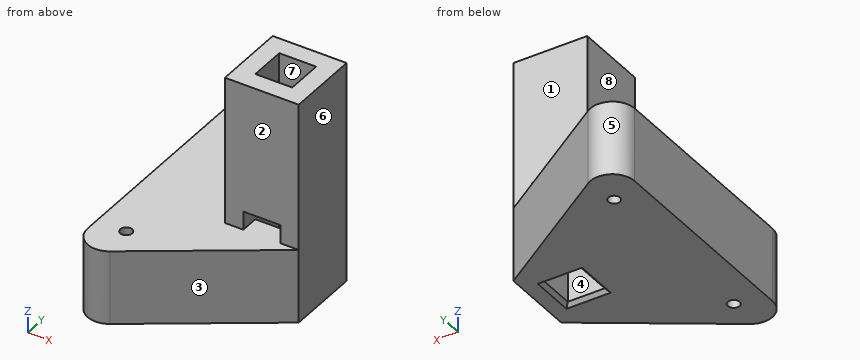
```python
from build123d import *

# Parameters (mm, degrees)
SKETCH_1_W          = 20
SKETCH_1_H          = 20
SKETCH_1_W_2        = 10
SKETCH_1_H_2        = 10
EXTRUDE_1_DEPTH     = 60
SKETCH_2_W          = 10
SKETCH_2_H          = 5
CUT_EXTRUDE_1_DEPTH = 80
SKETCH_4_R          = 1.6
EXTRUDE_3_DEPTH     = 20
CHAMFER_1_SIZE      = 1


with BuildPart() as part:
    # 草图1 → 凸台-拉伸1 (new body)
    with BuildSketch(Plane.XY):
        with Locations((5, 5)):
            Rectangle(SKETCH_1_W, SKETCH_1_H)
        with Locations((5, 5)):
            Rectangle(SKETCH_1_W_2, SKETCH_1_H_2, mode=Mode.SUBTRACT)
    extrude(amount=EXTRUDE_1_DEPTH)

    # 草图2 → 切除-拉伸1 (cut)
    with BuildSketch(Plane(origin=(0, 15, 0), x_dir=(1, 0, 0), z_dir=(0, 1, 0))):
        with Locations((5, -22.5)):
            Rectangle(SKETCH_2_W, SKETCH_2_H)
    extrude(amount=-CUT_EXTRUDE_1_DEPTH, mode=Mode.SUBTRACT)

    # 草图4 → 凸台-拉伸3 (add)
    with BuildSketch(Plane(origin=(0, 0, 0), x_dir=(-1, 0, 0), z_dir=(0, 0, -1))):
        with BuildLine():
            Line((30, 33.788897449), (30, -23.788897449))
            ThreePointArc((30, -23.788897449), (26.831147553, -29.078945042), (20.671798823, -28.781199215))
            Line((20.671798823, -28.781199215), (-15, -5))
            Line((-15, -5), (5, -5))
            Line((5, -5), (5, 15))
            Line((5, 15), (-15, 15))
            Line((-15, 15), (20.671798823, 38.781199215))
            ThreePointArc((20.671798823, 38.781199215), (26.831147553, 39.078945042), (30, 33.788897449))
        make_face()
        with Locations((22, -20)):
            Circle(SKETCH_4_R, mode=Mode.SUBTRACT)
        with Locations((22, 30)):
            Circle(SKETCH_4_R, mode=Mode.SUBTRACT)
    extrude(amount=-EXTRUDE_3_DEPTH)

    # 倒角1
    chamfer_1_edges = [part.edges().sort_by_distance(p)[0] for p in [
        (0, 5, 0),
        (5, 0, 0),
        (10, 5, 0),
        (5, 10, 0),
    ]]
    chamfer(chamfer_1_edges, length=CHAMFER_1_SIZE)


solid = part.part
```
Source: CAD feature listing. Evaluate the final solid. Frame: model axes, mm. Face numbers are marked on the shaded views. A direction names the side the tool comes from. Round coordinates to 2 decimals unless told otherwise and drop trailing zeros. Loops run counter-clockwise (first coordinate to the right, second up) from the corner with the lowest first, then second, coordinate; pieces in that order, holes last. Notation, with made-up numbers: M -37.75,24.5 L -8.75,24.5 A31 cw -8.75,57.5 Z; hole C 38,13 d5. An arc over 180 degrees is marked long. Put each result on its own line as item: value.
(1) Ray query, line 1 (Y direction, x = -22, z = 8); line 2 (Y direction, x = -22.5, z = 15.5); line 3 (Z direction, x = -24.5, y = -7). Return the intervals inside material, ascending. Write a range as [from, to].
Solutions:
line 1: [-29.45, -21.6], [-18.4, 28.4], [31.6, 39.45]
line 2: [-29.6, -21.52], [-18.48, 28.48], [31.52, 39.6]
line 3: [0, 20]
(2) Access query for the marked faces 1, 2, 3, 4 and 5. Directions: +Z, -Z, +X, -X, +Y, -Y. A direction counts if a zero-diameter tool reaches every point of the face in a straight line with its end or side. Return the directions, or none.
Solutions:
face 1: +Z, +X, -X, +Y
face 2: +Z, +X, -X, -Y
face 3: +Z, -Z, +X, -Y
face 4: +Z, -Z
face 5: +Z, -Z, +Y
(3) Section C-C, the plane x = -22. Return loops of the section in (y, z).
Solutions:
outline: M -29.45,0 L -21.6,0 L -21.6,20 L -29.45,20 Z; M -18.4,0 L 28.4,0 L 28.4,20 L -18.4,20 Z; M 31.6,0 L 39.45,0 L 39.45,20 L 31.6,20 Z
(4) First-contact query: pin 1 (16 mm diameter, centred on x = 7, z = 43.5, fed in from +Y); pin 2 (22 mm diameter, centred on x = 9.5, z = 46, fed in from -Y); pin 3 (1.5 mm diameter, centred on x = 6, z = 18.5, fed in from -Y); pin 4 (1.5 mm diameter, centred on x = 4.5, y = 8, fed in from +Z). Flat tips, straight axial feed; report the tip coordinate or a pass-through.
Solutions:
pin 1: y = 15
pin 2: y = -5
pin 3: y = -11.5
pin 4: through
(5) Section D-D, the plane z = 19. Return loops of the section in (x, y), and give its area (3 significant figures).
Solutions:
outline: M -30,-23.79 A6 ccw -20.67,-28.78 L 15,-5 L 15,15 L -20.67,38.78 A6 ccw -30,33.79 Z; hole C -22,-20 d3.2; hole C -22,30 d3.2; hole M 0,0 L 10,0 L 10,10 L 0,10 Z
area: 2,080 mm²
(6) Section B-B, the plane z = 45. Return loops of the section in (x, y), and give its area (3 significant figures).
Solutions:
outline: M -5,-5 L 15,-5 L 15,15 L -5,15 Z; hole M 0,0 L 10,0 L 10,10 L 0,10 Z
area: 300 mm²
(7) Pull-direction query (X, two-part tool) for the marked faces 6, 7 and 8; classes: released by +X, released by -X, zero draft, split by the parting line, or undercut.
Solutions:
face 6: released by +X
face 7: undercut
face 8: released by -X
(8) Section A-A, the plane y = 30. Return loops of the section in (x, z).
Solutions:
outline: M -30,0 L -23.6,0 L -23.6,20 L -30,20 Z; M -20.4,0 L -7.5,0 L -7.5,20 L -20.4,20 Z
